Autodesk Inventor part; units mm, degrees
ref_plane "YZ Plane" through (0, 0, 0) normal (1, 0, 0) x (0, 1, 0)
ref_plane "XZ Plane" through (0, 0, 0) normal (0, 1, 0) x (-1, 0, 0)
ref_plane "XY Plane" through (0, 0, 0) normal (0, 0, 1) x (1, 0, 0)
sketch "スケッチ1" plane through (0, 0, 0) normal (0, 0, 1) x (1, 0, 0)
  line L0 (0, 0) -> (20, 0)
  line L1 (20, 0) -> (20, 20)
  line L2 (20, 20) -> (0, 20)
  line L3 (0, 20) -> (0, 0)
  line L4 (0, 10) -> (20, 10) construction
  circle A0 centre (5, 10) radius 1.75
  line L5 (10, 20) -> (10, 0) construction
  circle A1 centre (15, 10) radius 1.75
  dimension "d0" = 20
  dimension "d1" = 20
  dimension "d2" = 10
  dimension "d3" = 3.5
  dimension "d4" = 10
extrude "押し出し1" add sketch "スケッチ1" along normal blind 6
sketch "スケッチ2" plane through (0, 0, 0) normal (0, -1, 0) x (1, 0, 0)
  line L0 (0, 0) -> (20, 0) construction
  line L1 (10, 0) -> (10, 6) construction
  line L2 (0, 6) -> (20, 6) construction
  line L3 (7.5, 6) -> (8.091, 4.1087)
  line L4 (11.909, 4.1087) -> (12.5, 6)
  line L5 (7.5, 6) -> (12.5, 6)
  arc A0 (8.091, 4.1087) -> (11.909, 4.1087) centre (10, 4.7052) ccw
  point P0 (10, -2)
  dimension "d11" = 2
  dimension "d18" = 5
  dimension "d19" = 8
extrude "押し出し2" cut sketch "スケッチ2" against normal through all
chamfer "面取り1" distance 6 angle 45 4 edges at (20, 20, 3) (0, 20, 3) (20, 0, 3) (0, 0, 3)
properties part number "_3D プリント"
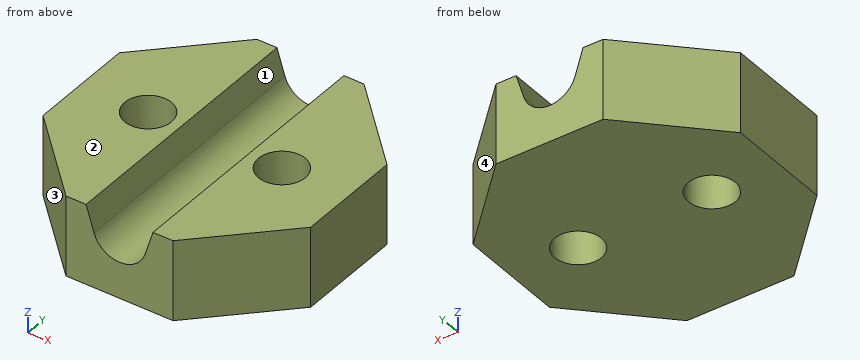
Here's how the part is built. I have some questions about the finished solid (model axes, mm). Face numbers are marked on the shaded views. Give positions to 0.01 mm unless a question says otherwise; leave off trailing zeros. Order: outer loops, then holes, each group sorted by start corner. A loop starts at its lowest first (then second) coordinate and runs counter-clockwise, first axis right, second up. Notation, with made-up numbers: (-18, -33.75) -> (24, -33.75) arc R17 ccw to (24, -14.75) -> close; hole circle Ø4 at (-1.5, 50.5). An arc over 180 degrees is marked (long way). One line per item, written item: value. Start each with the question number.
1. Imagine slicing it at C-C, the plane z = 1.5. List the corners of the cut face in (x, y) for me.
2. Will this pin go through, and if not, where does the flat tip stop? pin 1 Ø3 at (x, z) = (3, 5) entering from +Y.
3. Imagine slicing it at D-D, the plane y = 17.5. List the corners of the cut face in (x, z) for me, plus the area to 3 significant figures.
4. We'd pull the mould along X, two halves only. Please class the marked faces 1, 2, 3 and 4: released by +X, released by -X, zero draft, split by the parting line, or undercut.
5. I need wall thicknesses on probe 1 along X at (y, z) = (10.5, 3); probe 2 along Y at (x, z) = (14.75, 4.75); probe 3 along X at (y, z) = (7.5, 4.25). Which ranges of each line are inside material? Lowest first, please. Write a range as from..to.
6. Imagine slicing it at B-B, the plane y = 10. List the corners of the cut face in (x, z) for me.
7. Imagine slicing it at A-A, the plane x = 5. List the corners of the cut face in (y, z) for me, plus the area to 3 significant figures.
Values follow:
1. outline: (0, 6) -> (6, 0) -> (14, 0) -> (20, 6) -> (20, 14) -> (14, 20) -> (6, 20) -> (0, 14) -> close; hole circle Ø3.5 at (5, 10); hole circle Ø3.5 at (15, 10)
2. pin 1: stops at y = 18.5
3. outline: (3.5, 0) -> (16.5, 0) -> (16.5, 6) -> (12.5, 6) -> (11.91, 4.11) arc R2 cw to (8.09, 4.11) -> (7.5, 6) -> (3.5, 6) -> close
3. area: 65.7 mm2
4. face 1: undercut
4. face 2: zero draft
4. face 3: released by -X
4. face 4: released by +X
5. probe 1: x = 0..3.32, 6.68..8.95, 11.05..13.32, 16.68..20
5. probe 2: y = 0.75..8.27, 11.73..19.25
5. probe 3: x = 0..8.05, 11.95..20
6. outline: (0, 0) -> (3.25, 0) -> (3.25, 6) -> (0, 6) -> close; (6.75, 0) -> (13.25, 0) -> (13.25, 6) -> (12.5, 6) -> (11.91, 4.11) arc R2 cw to (8.09, 4.11) -> (7.5, 6) -> (6.75, 6) -> close; (16.75, 0) -> (20, 0) -> (20, 6) -> (16.75, 6) -> close
7. outline: (1, 0) -> (8.25, 0) -> (8.25, 6) -> (1, 6) -> close; (11.75, 0) -> (19, 0) -> (19, 6) -> (11.75, 6) -> close
7. area: 87.0 mm2
